Source: CAD feature listing. Evaluate the final solid. Frame: model axes, mm. Give positions to 0.01 mm unless a question says otherwise; leave off trailing zeros. Write each loop counter-clockwise with the first axis right and the second up, starting at its lowest first coordinate (ties: lowest second). Pieces come first, ordered by that corner, then holes. Notation, with made-up numbers: (60, 63) - (88, 63) arc R16 ccw to (88, 74) - close; hole circle Ø11 at (62.5, 59). An arc over 180 degrees is marked (long way). One line per question, with ' | ' between items. Start each with the question number.
(1) Section B-B, the plane x = 7.5. Return loops of the section in (y, z) (3 decimals), plus the area to 3 significant figures.
(2) Section A-A, the plane y = 10.25. Return loops of the section in (x, z) (3 decimals), plus the area to 3 significant figures.
(3) Pin query (flat end, axial travel): pin 1 (5 mm diameter, centred on x = 14.5, y = 6.5, fed in from -Z). Return the tip coordinate at first contact, or that it passes through.
(4) Ray query, line 1 (X direction, y = 10, z = 1.85); line 2 (X direction, y = 7.25, z = 0.35); line 3 (X direction, y = 16.5, z = 1.6). Return the intervals inside material, ascending. Write a range as [from, to].
(5) Section D-D, the plane y = 2.5. Return loops of the section in (x, z) (3 decimals).
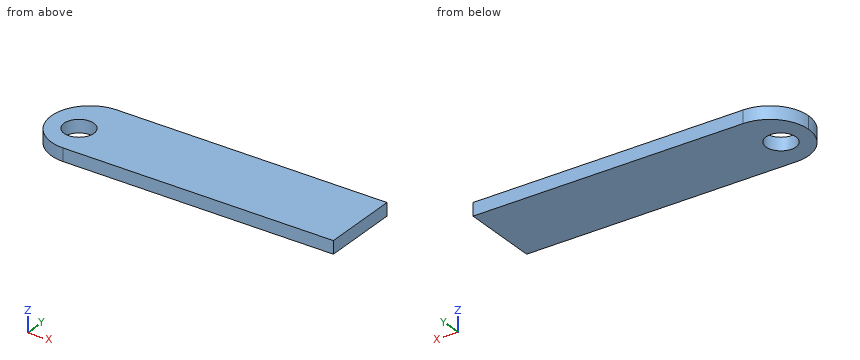
```python
from build123d import *

# Parameters (mm, degrees)
SKETCH1_W           = 76.2
SKETCH1_H           = 19.05
BOSS_EXTRUDE1_DEPTH = 3.175
FILLET1_R           = 9.525
SKETCH2_R           = 3.683
CUT_EXTRUDE1_DEPTH  = 79.60930686


with BuildPart() as part:
    # Sketch1 → Boss-Extrude1 (new body)
    with BuildSketch(Plane.XY):
        with Locations((38.1, 9.525)):
            Rectangle(SKETCH1_W, SKETCH1_H)
    extrude(amount=BOSS_EXTRUDE1_DEPTH)

    # Fillet1
    fillet1_edges = [part.edges().sort_by_distance(p)[0] for p in [
        (0, 0, 1.5875),
        (0, 19.05, 1.5875),
    ]]
    fillet(fillet1_edges, radius=FILLET1_R - 0.0001)  # a hair under: the kernel refuses the full size

    # Sketch2 → Cut-Extrude1 (cut, through all)
    with BuildSketch(Plane.XY.offset(3.175)):
        with Locations((7.553506199, 8.47367626)):
            Circle(SKETCH2_R)
    extrude(amount=-CUT_EXTRUDE1_DEPTH, mode=Mode.SUBTRACT)


solid = part.part
```
Check sheet entries:
1) outline: (0.218, 0) - (4.791, 0) - (4.791, 3.175) - (0.218, 3.175) - close; (12.156, 0) - (18.832, 0) - (18.832, 3.175) - (12.156, 3.175) - close | area: 35.7 mm²
2) outline: (0.028, 0) - (4.327, 0) - (4.327, 3.175) - (0.028, 3.175) - close; (10.78, 0) - (76.2, 0) - (76.2, 3.175) - (10.78, 3.175) - close | area: 221 mm²
3) pin 1: z = 0
4) line 1: [0.01, 4.2], [10.91, 76.2] | line 2: [0.28, 4.08], [11.03, 76.2] | line 3: [3.04, 76.2]
5) outline: (3.093, 0) - (76.2, 0) - (76.2, 3.175) - (3.093, 3.175) - close
